Check sheet for the modelled part. Datum: model origin and axes. Units: mm. Face numbers are marked on the shaded views. A direction names the side the tool comes from. Give positions to 0.01 mm unless a question says otherwise; leave off trailing zeros. Loops run counter-clockwise (first coordinate to the right, second up) from the corner with the lowest first, then second, coordinate; pieces in that order, holes last. Notation, with made-up numbers: M 86,63.25 L 118,63.25 A35 cw 118,97.25 Z; hole C 33,-9 d2. An arc over 180 degrees is marked long. Use one line per item in the form item = value.
from build123d import *

# Parameters (mm, degrees)
BOSS_EXTRUDE1_DEPTH = 5
SKETCH2_R           = 0.5
CUT_EXTRUDE1_DEPTH  = 5
CUT_EXTRUDE2_DEPTH  = 1
CUT_EXTRUDE3_DEPTH  = 2


with BuildPart() as part:
    # Sketch1 → Boss-Extrude1 (new body)
    with BuildSketch(Plane.XY):
        with BuildLine():
            Line((-5, 0), (-3, 0))
            ThreePointArc((-3, 0), (0, 3), (3, 0))
            Line((3, 0), (5, 0))
            ThreePointArc((5, 0), (0, 5), (-5, 0))
        make_face()
    extrude(amount=BOSS_EXTRUDE1_DEPTH)

    # Sketch2 → Cut-Extrude1 (cut)
    with BuildSketch(Plane(origin=(0, 0, 0), x_dir=(1, 0, 0), z_dir=(0, 1, 0))):
        with Locations((0, -1)):
            Circle(SKETCH2_R)
        Polygon((-5, -1), (-4.001262059, -1), (-4.001262059, -1.997514784), (-4.001262059, -2.994544778), (0, -2.994544778), (0, -5), (-5, -5), align=None)
    extrude(amount=CUT_EXTRUDE1_DEPTH, mode=Mode.SUBTRACT)

    # Sketch3 → Cut-Extrude2 (cut)
    with BuildSketch(Plane.XY.offset(5)):
        with BuildLine():
            Line((0, 4), (0, 0))
            Line((0, 0), (4, 0))
            ThreePointArc((4, 0), (2.828427125, 2.828427125), (0, 4))
        make_face()
    extrude(amount=-CUT_EXTRUDE2_DEPTH, mode=Mode.SUBTRACT)

    # Sketch4 → Cut-Extrude3 (cut)
    with BuildSketch(Plane.XY.offset(2.994544778)):
        with BuildLine():
            Line((-3.001262059, 3), (-3.001262059, 3.999053144))
            ThreePointArc((-3.001262059, 3.999053144), (-4.472488697, 2.235362354), (-5, 0))
            Line((-5, 0), (-4.001262059, 0))
            ThreePointArc((-4.001262059, 0), (-3.811157575, 1.603298505), (-3.001262059, 3))
        make_face()
    extrude(amount=-CUT_EXTRUDE3_DEPTH, mode=Mode.SUBTRACT)


solid = part.part
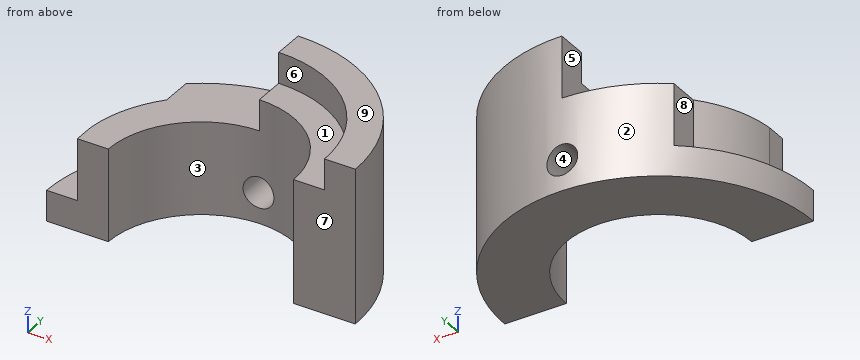
1) Section check A-A (y = 1.1). Record the cut outline in (x, z), then the cut area to 3 significant figures.
Evaluation:
outline = M -4.88,0 L -2.79,0 L -2.79,2.99 L -3.94,2.99 L -3.94,0.99 L -4.88,0.99 Z; M 2.79,0 L 4.88,0 L 4.88,5 L 3.85,5 L 3.85,4 L 2.79,4 Z
area = 13.8 mm^2
2) Scan lines: line 1 (Z direction, x = -4.25, y = 0.95); line 2 (Z direction, x = 1, y = 3.5); line 3 (Y direction, x = 4, z = 2.95). Record each from-to range of solid material in increasing order.
Evaluation:
line_1 = 0 to 0.99
line_2 = 0 to 4
line_3 = 0 to 3
3) Release check for a two-part mould opening along X. For the marked faces 1, 2, 3 and 4 record: pulls with the +X half, pulls with the -X half, needs draft (parallel to the pull), parting line crosses it, or undercut.
Evaluation:
face_1 = needs draft
face_2 = parting line crosses it
face_3 = undercut
face_4 = undercut
4) Section check C-C (x = -3.25). Record the cut outline in (y, z).
Evaluation:
outline = M 0,0 L 3.8,0 L 3.8,0.99 L 2.69,0.99 L 2.69,2.99 L 0,2.99 Z
5) Depth check by flat-ended pin: pin 1 Ø1.2 at (x, y) = (-1, 3) entering from +Z; pin 2 Ø1.5 at (y, z) = (0.5, 1) entering from +X; pin 3 Ø0.6 at (y, z) = (4, 4) entering from -X; pin 4 Ø0.5 at (y, z) = (3.5, 1.5) entering from -X. Enter the tip coordinate at first touch or a pass-through.
Evaluation:
pin_1 = 2.99
pin_2 = 5
pin_3 = 0
pin_4 = -3
6) Section check D-D (y = 2). Record the cut outline in (x, z).
Evaluation:
outline = M -4.58,0 L -2.24,0 L -2.24,2.99 L -3.65,2.99 L -3.65,0.99 L -4.58,0.99 Z; M 2.24,0 L 4.58,0 L 4.58,5 L 3.46,5 L 3.46,4 L 2.24,4 Z
7) Section check B-B (z = 2.45). Record the cut outline in (x, y).
Evaluation:
outline = M -4,0 L -3,0 A3 cw 3,0 L 5,0 A5 ccw -3,4 L -3,3 A3.99 ccw -4,0.68 Z
8) Set-up check for the marked faces 5, 6, 7, 8 and 9: record each of +Z, -Z, +X, -X, +Y, -Y from which the full face is reachable in a straight line by a thin tool's end or side.
Evaluation:
face_5 = +Z, -X, +Y, -Y
face_6 = +Z, -X, -Y
face_7 = +Z, -Z, +X, -X, -Y
face_8 = +Z, -X, +Y
face_9 = +Z, +X, -X, +Y, -Y
